Check sheet for the modelled part. Datum: model origin and axes. Units: mm. A direction names the side the tool comes from. Give positions to 0.01 mm unless a question says otherwise; leave off trailing zeros. Use a Markdown table: item, result. Add a question column.
1. Cross-section at A-A (y = 340.5). Count the separate pieces of the cut face and the enclosed holes in it, then the cut area to 3 significant figures.
2. Scan lines: probe 1 along Z at (x, y) = (-694, 202.5); probe 2 along X at (y, z) = (266.5, 24); probe 3 along Y at (x, z) = (-729, 5). Record each from-to range of solid material in increasing order. Write a range as [from, to].
3. Set-up check for faces 1 (the flat face through (-972.075, 218, 27)), 2 (the flat face through (-972.075, 220, -12)), 3 (the cylindrical face through (-953.56, 363.05, 7.6)): record each of +Z, -Z, +X, -X, +Y, -Y from which the full face is reachable in a straight line by a thin tool's end or side.
4. Gauge pin test, flat ends, axial feed: P1, Ø6.5, axis at y = 163.12, z = 7.5, coming from the +X side; P2, Ø12, axis at x = -451.5, y = 212.5, coming from the +Z side; P3, Ø12.5, axis at y = 235.5, z = -15.5, coming from the +X side; P4, Ø5, axis at x = -266, y = 257.5, coming from the +Z side. Record the tip position at first contact, or that the pin passes through.
from build123d import *

# Parameters (mm, degrees)
F0_W      = 1200
F0_H      = 250
F1_DEPTH  = 15
F3_DEPTH  = 25
F4_R      = 100
F6_D      = 8
F6_DEPTH  = 60
F6_TIP    = 2.4034424761
F8_D      = 8
F8_DEPTH  = 60
F8_TIP    = 2.4034424761
F9_R      = 55
F10_DEPTH = 25
F12_DEPTH = 25
F14_DEPTH = 25


# Not quite as in the source:
# - a feature names something its author has since deleted; it is built from what else it names


with BuildPart() as f1:
    # F0 (on Top) → F1 (new body)
    with BuildSketch(Plane.XY):
        with Locations((-382.0752739906, 268.1212723255)):
            Rectangle(F0_W, F0_H)
    extrude(amount=F1_DEPTH)

    # F2 (on face) → F3 (cut)
    with BuildSketch(Plane.XY.offset(15)):
        with BuildLine():
            add(Edge.make_bspline(
                [(-982.0752739906, 143.1212723255), (-381.1290302773, 253.1212723255), (-296.0948119124, 253.1212723255), (217.9247260094, 143.1212723255)],
                knots=[0, 0, 0, 0, 1200, 1200, 1200, 1200], degree=3))
            Line((-982.0752739906, 143.1212723255), (217.9247260094, 143.1212723255))
        make_face()
    extrude(amount=-F3_DEPTH, mode=Mode.SUBTRACT)

    # F4
    f4_edges = [f1.edges().sort_by_distance(p)[0] for p in [
        (-982.075274, 393.121272, 7.5),
        (217.924726, 393.121272, 7.5),
    ]]
    fillet(f4_edges, radius=F4_R)

    # F6
    with Locations(Plane(origin=(-982.0752739906, 0, 0), x_dir=(0, -1, 0), z_dir=(-1, 0, 0))):
        with Locations((-163.1212723255, 7.5), (-213.1212723255, 7.5), (-263.1212723255, 7.5)):
            Hole(F6_D / 2, depth=F6_DEPTH)
            with Locations((0, 0, -(F6_DEPTH + F6_TIP / 2))):  # 118° drill point
                Cone(0, F6_D / 2, F6_TIP, mode=Mode.SUBTRACT)

    # F8
    with Locations(Plane.YZ.offset(217.9247260094)):
        with Locations((163.1212723255, 7.5), (213.1212723255, 7.5), (263.1212723255, 7.5)):
            Hole(F8_D / 2, depth=F8_DEPTH)
            with Locations((0, 0, -(F8_DEPTH + F8_TIP / 2))):  # 118° drill point
                Cone(0, F8_D / 2, F8_TIP, mode=Mode.SUBTRACT)

    # F9 (on face) → F10 (cut)
    with BuildSketch(Plane.XY.offset(15)):
        with Locations((-902.0752739906, 308.2580530366)):
            Circle(F9_R)
        with Locations((-772.0752739906, 308.2580530366)):
            Circle(F9_R)
        with Locations((-642.0752739906, 308.2580530366)):
            Circle(F9_R)
        with Locations((-512.0752739906, 308.2580530366)):
            Circle(F9_R)
        with Locations((-382.0752739906, 308.2580530366)):
            Circle(F9_R)
        with Locations((-252.0752739906, 308.2580530366)):
            Circle(F9_R)
        with Locations((-122.0752739906, 308.2580530366)):
            Circle(F9_R)
        with Locations((7.9247260094, 308.2580530366)):
            Circle(F9_R)
        with Locations((137.9247260094, 308.2580530366)):
            Circle(F9_R)
    extrude(amount=-F10_DEPTH, mode=Mode.SUBTRACT)

    # F11 (on face) → F12 (join)
    with BuildSketch(Plane(origin=(0, 0, 0), x_dir=(1, 0, 0), z_dir=(0, 0, -1))):
        with BuildLine():
            add(Edge.make_bspline(
                [(-972.0752739906, -144.9502384932), (-973.3234960268, -144.7221332236), (-974.5722289185, -144.4938787017), (-975.8214712324, -144.265475917), (-977.0712215354, -144.0369258537), (-978.3214783948, -143.8082294911), (-979.5722403783, -143.5793878034), (-980.823506054, -143.3504017601), (-982.0752739906, -143.1212723255)],
                knots=[0.9928997665, 0.9928997665, 0.9928997665, 0.9928997665, 0.9928997665, 0.9928997665, 0.9928997665, 0.9928997665, 0.9928997665, 1, 1, 1, 1, 1, 1, 1, 1, 1], degree=8))
            Line((-982.0752739906, -143.1212723255), (-982.0752739906, -293.1212723255))
            Line((-982.0752739906, -293.1212723255), (-972.0752739906, -293.1212723255))
            Line((-972.0752739906, -293.1212723255), (-972.0752739906, -144.9502384932))
        make_face()
    extrude(amount=F12_DEPTH)

    # F13 (on face) → F14 (join)
    with BuildSketch(Plane.XY.offset(15)):
        with BuildLine():
            Line((-982.0752739906, 293.1212723255), (-982.0752739906, 143.1212723255))
            add(Edge.make_bspline(
                [(-982.0752739906, 143.1212723255), (-978.7259696098, 143.7343446023), (-975.3926908046, 144.3439999918), (-972.0752739906, 144.9502384937)],
                knots=[0, 0, 0, 0, 6.6880612018, 6.6880612018, 6.6880612018, 6.6880612018], degree=3))
            Line((-972.0752739906, 144.9502384937), (-972.0752739906, 293.1212723255))
            Line((-972.0752739906, 293.1212723255), (-982.0752739906, 293.1212723255))
        make_face()
    extrude(amount=F14_DEPTH)


solid = f1.part
Worked answers:
| question | item | result |
|---|---|---|
| 1 | separate pieces | 10 |
| 1 | enclosed holes | 0 |
| 1 | area | 5,610 mm² |
| 2 | probe 1 | z = [0, 15] |
| 2 | probe 2 | x = [-982.08, -972.08] |
| 2 | probe 3 | y = [187.53, 274.06], [342.46, 393.12] |
| 3 | face 1 | +Z, +X, +Y, -Y |
| 3 | face 2 | -Z, +X, +Y, -Y |
| 3 | face 3 | +Z, -Z, -X, +Y |
| 4 | P1 | stops at x = 157.47 |
| 4 | P2 | passes through |
| 4 | P3 | stops at x = -972.08 |
| 4 | P4 | stops at z = 15 |
